```python
from build123d import *

# Parameters (mm, degrees)
BOX001_W         = 10
BOX001_H         = 110
BOX001_DEPTH     = 10
ARRAY001_X_COUNT = 4
ARRAY001_X_PITCH = 20
BOX_W            = 110
BOX_H            = 10
BOX_DEPTH        = 10
ARRAY_Y_COUNT    = 4
ARRAY_Y_PITCH    = 20
BOX003_W         = 70
BOX003_H         = 70
BOX003_DEPTH     = 130
BOX002_W         = 90
BOX002_H         = 90
BOX002_DEPTH     = 150


with BuildPart() as array001:
    # Box001 → Box001 (new body)
    with BuildSketch(Plane.XY):
        with Locations((5, 55)):
            Rectangle(BOX001_W, BOX001_H)
    extrude(amount=BOX001_DEPTH)

    # Array001 X: Array001 ×4


with BuildPart() as array001_1:
    add(array001.part)
    with Locations(*[(i * ARRAY001_X_PITCH, 0, 0) for i in range(1, ARRAY001_X_COUNT)]):
        add(array001.part)


with BuildPart() as array001_2:
    # Array001 placement: moved
    add(array001_1.part.moved(Location((20, -20, 0))))


with BuildPart() as fusion:
    # Box → Box (new body)
    with BuildSketch(Plane.XY):
        with Locations((55, 5)):
            Rectangle(BOX_W, BOX_H)
    extrude(amount=BOX_DEPTH)

    # Array Y: Fusion ×4


with BuildPart() as fusion_1:
    add(fusion.part)
    with Locations(*[(0, i * ARRAY_Y_PITCH, 0) for i in range(1, ARRAY_Y_COUNT)]):
        add(fusion.part)

    # Fusion: union Array001
    add(array001_2.part)


with BuildPart() as fusion_2:
    # Fusion placement: moved
    add(fusion_1.part.moved(Location((-10, 10, 140))))


with BuildPart() as cub003:
    # Box003 → Box003 (new body)
    with BuildSketch(Plane(origin=(10, 10, 20), x_dir=(1, 0, 0), z_dir=(0, 0, 1))):
        with Locations((35, 35)):
            Rectangle(BOX003_W, BOX003_H)
    extrude(amount=BOX003_DEPTH)


with BuildPart() as cut001:
    # Box002 → Box002 (new body)
    with BuildSketch(Plane.XY):
        with Locations((45, 45)):
            Rectangle(BOX002_W, BOX002_H)
    extrude(amount=BOX002_DEPTH)

    # Cut: cut Cub003
    add(cub003.part, mode=Mode.SUBTRACT)

    # Cut001: cut Fusion
    add(fusion_2.part, mode=Mode.SUBTRACT)


solid = cut001.part
```
Check sheet for the modelled part. Datum: model origin and axes. Units: mm. A direction names the side the tool comes from. Coordinates: 2 decimals unless noted, no trailing zeros. Write each loop counter-clockwise with the first axis right and the second up, starting at its lowest first coordinate (ties: lowest second). Pieces come first, ordered by that corner, then holes. Notation, with made-up numbers: (32.5, 19.25) -> (63.5, 19.25) arc R36 cw to (63.5, 53.25) -> close; hole circle Ø7 at (-21, 2.5). An arc over 180 degrees is marked (long way). Use a Markdown table: item, result.
1. Sectioned sample at A-A (y = 7). Enter the section's corners in (x, z), plus the area to 3 significant figures.
Reported:
| item | result |
|---|---|
| outline | (0, 0) -> (90, 0) -> (90, 150) -> (80, 150) -> (80, 140) -> (70, 140) -> (70, 150) -> (60, 150) -> (60, 140) -> (50, 140) -> (50, 150) -> (40, 150) -> (40, 140) -> (30, 140) -> (30, 150) -> (20, 150) -> (20, 140) -> (10, 140) -> (10, 150) -> (0, 150) -> close |
| area | 13,100 mm2 |
2. Sectioned sample at C-C (x = 38). Enter the section's corners in (y, z), plus the area to 3 significant figures.
Reported:
| item | result |
|---|---|
| outline | (0, 0) -> (90, 0) -> (90, 140) -> (80, 140) -> (80, 20) -> (10, 20) -> (10, 140) -> (0, 140) -> close |
| area | 4,200 mm2 |
3. Release check for a two-part mould opening along X. For faces 6 (the flat face through (40, 5, 145)), 7 (the flat face through (25, 85, 150)), 8 (the flat face through (15, 85, 140)) record: pulls with the +X half, pulls with the -X half, needs draft (parallel to the pull), parting line crosses it, or undercut.
Reported:
| item | result |
|---|---|
| face 6 | undercut |
| face 7 | needs draft |
| face 8 | undercut |
4. Sectioned sample at D-D (y = 22). Enter the section's corners in (x, z), plus the area to 3 significant figures.
Reported:
| item | result |
|---|---|
| outline | (0, 0) -> (90, 0) -> (90, 150) -> (80, 150) -> (80, 20) -> (10, 20) -> (10, 150) -> (0, 150) -> close |
| area | 4,400 mm2 |
5. Go/stop test with flat-tipped pins: pin 1 Ø5 at (x, y) = (36.5, 86.5) entering from +Z; pin 2 Ø5 at (x, y) = (52, 16) entering from +Z. Record where each tip stops, or that it passes through.
Reported:
| item | result |
|---|---|
| pin 1 | stops at z = 140 |
| pin 2 | stops at z = 20 |
6. Sectioned sample at B-B (z = 107). Enter the section's corners in (x, y).
Reported:
| item | result |
|---|---|
| outline | (0, 0) -> (90, 0) -> (90, 90) -> (0, 90) -> close; hole (10, 10) -> (80, 10) -> (80, 80) -> (10, 80) -> close |
7. Scan lines: line 1 along Y through (x, z) = (29.5, 31.5); line 2 along Z through (x, y) = (62, 22.5). Record each from-to range of solid material in increasing order.
Reported:
| item | result |
|---|---|
| line 1 | y = 0 to 10, 80 to 90 |
| line 2 | z = 0 to 20 |
8. Tool access check on faces 1 (the flat face through (45, 10, 84)), 2 (the flat face through (5, 70, 145)), 3 (the flat face through (85, 65, 150)), 4 (the flat face through (60, 85, 145)), 5 (the flat face through (44, 46, 0)). Record the directions out of +Z, -Z, +X, -X, +Y, -Y that give a thin tool (end or side, any length) a straight path to the whole face; none if there is none.
Reported:
| item | result |
|---|---|
| face 1 | +Z |
| face 2 | +Z, +X, -X |
| face 3 | +Z, +X, -X, +Y, -Y |
| face 4 | +Z, +Y, -Y |
| face 5 | -Z, +X, -X, +Y, -Y |
